from build123d import *

# Parameters (mm, degrees)
F0_R     = 16.25
F1_DEPTH = 9
F2_D     = 3.2
F2_DEPTH = 40


with BuildPart() as f1:
    # F0 (on Top) → F1 (new body)
    with BuildSketch(Plane.XY):
        with BuildLine():
            ThreePointArc((13.85, -17.413788), (20.040272, -9.666954), (22.25, 0))
            ThreePointArc((22.25, 0), (22.075626, 2.780148), (21.555238, 5.51672))
            Line((21.555238, 5.51672), (19.324579, 4.228848))
            Line((19.324579, 4.228848), (13.324579, 14.621152))
            Line((13.324579, 14.621152), (15.555238, 15.909024))
            ThreePointArc((15.555238, 15.909024), (14.721858, 16.683207), (13.85, 17.413788))
            Line((13.85, 17.413788), (-13.85, 17.413788))
            ThreePointArc((-13.85, 17.413788), (-22.25, 0), (-13.85, -17.413788))
            Line((-13.85, -17.413788), (13.85, -17.413788))
        make_face()
        Circle(F0_R, mode=Mode.SUBTRACT)
        with BuildLine():
            ThreePointArc((-8.031189, -20.75), (-11.067032, -19.302417), (-13.85, -17.413788))
            Line((-13.85, -17.413788), (-13.85, -28.75))
            Line((-13.85, -28.75), (-10.25, -28.75))
            Line((-10.25, -28.75), (-10.25, -20.75))
            Line((-10.25, -20.75), (-8.031189, -20.75))
        make_face()
        with BuildLine():
            ThreePointArc((8.031189, -20.75), (11.067032, -19.302417), (13.85, -17.413788))
            Line((13.85, -17.413788), (-13.85, -17.413788))
            ThreePointArc((-13.85, -17.413788), (-11.067032, -19.302417), (-8.031189, -20.75))
            Line((-8.031189, -20.75), (8.031189, -20.75))
        make_face()
        with BuildLine():
            Line((13.85, -28.75), (13.85, -17.413788))
            ThreePointArc((13.85, -17.413788), (11.067032, -19.302417), (8.031189, -20.75))
            Line((8.031189, -20.75), (10.25, -20.75))
            Line((10.25, -20.75), (10.25, -28.75))
            Line((10.25, -28.75), (13.85, -28.75))
        make_face()
        with BuildLine():
            ThreePointArc((8.031189, 20.75), (11.067032, 19.302417), (13.85, 17.413788))
            Line((13.85, 17.413788), (13.85, 28.75))
            Line((13.85, 28.75), (10.25, 28.75))
            Line((10.25, 28.75), (10.25, 20.75))
            Line((10.25, 20.75), (8.031189, 20.75))
        make_face()
        with BuildLine():
            Line((-13.85, 17.413788), (13.85, 17.413788))
            ThreePointArc((13.85, 17.413788), (11.067032, 19.302417), (8.031189, 20.75))
            Line((8.031189, 20.75), (-8.031189, 20.75))
            ThreePointArc((-8.031189, 20.75), (-11.067032, 19.302417), (-13.85, 17.413788))
        make_face()
        with BuildLine():
            Line((-13.85, 28.75), (-13.85, 17.413788))
            ThreePointArc((-13.85, 17.413788), (-11.067032, 19.302417), (-8.031189, 20.75))
            Line((-8.031189, 20.75), (-10.25, 20.75))
            Line((-10.25, 20.75), (-10.25, 28.75))
            Line((-10.25, 28.75), (-13.85, 28.75))
        make_face()
    extrude(amount=F1_DEPTH)

    # F2
    with Locations(Plane(origin=(0, 0, 0), x_dir=(1, 0, 0), z_dir=(0, 0, -1))):
        with Locations((-9.625, -16.670989), (9.625, -16.670989), (19.25, 0), (9.625, 16.670989), (-9.625, 16.670989), (-19.25, 0)):
            Hole(F2_D / 2, depth=F2_DEPTH)


solid = f1.part
The listing builds one solid part. Answer for the finished solid, in the listing's coordinates (mm). A direction names the side the tool comes from. Coordinates: 2 decimals unless noted, no trailing zeros. Write each loop counter-clockwise with the first axis right and the second up, starting at its lowest first coordinate (ties: lowest second). Pieces come first, ordered by that corner, then holes. Notation, with made-up numbers: (50, 48) - (96, 48) arc R14 cw to (96, 63) - close; hole circle Ø3 at (49.5, 74.5). An arc over 180 degrees is marked (long way). Put each result on its own line as item: value.
1. The part is cut by section A-A on x = 0. Give the vertices of the cut face in (y, z), plus the area to 3 significant figures.
Answer sheet:
outline: (-20.75, 0) - (-16.25, 0) - (-16.25, 9) - (-20.75, 9) - close; (16.25, 0) - (20.75, 0) - (20.75, 9) - (16.25, 9) - close
area: 81.0 mm^2
2. The part is cut by section C-C on z = 7.5. Give the vertices of the cut face in (x, y) (3 decimals).
Answer sheet:
outline: (-13.85, -28.75) - (-10.25, -28.75) - (-10.25, -20.75) - (10.25, -20.75) - (10.25, -28.75) - (13.85, -28.75) - (13.85, -17.414) arc R22.25 ccw to (22.25, 0) arc R22.25 ccw to (21.555, 5.517) - (19.325, 4.229) - (13.325, 14.621) - (15.555, 15.909) arc R22.25 ccw to (13.85, 17.414) - (13.85, 28.75) - (10.25, 28.75) - (10.25, 20.75) - (-10.25, 20.75) - (-10.25, 28.75) - (-13.85, 28.75) - (-13.85, 17.414) arc R22.25 ccw to (-13.85, -17.414) - close; hole circle Ø3.2 at (-19.25, 0); hole circle Ø32.5 at (0, 0); hole circle Ø3.2 at (-9.625, -16.671); hole circle Ø3.2 at (-9.625, 16.671); hole circle Ø3.2 at (9.625, -16.671); hole circle Ø3.2 at (9.625, 16.671); hole circle Ø3.2 at (19.25, 0)
3. A tool of negligible diameter and unlimited length cuts with its end or side. For faces 4 (the face through (-13.85, 23, 4)), 5 (the face through (13.85, 23, 4)), 6 (the face through (10.25, -25, 4)), from which of +Z, -Z, +X, -X, +Y, -Y can it reach the whole face along a straight path? Write none if from no direction.
Answer sheet:
face 4: +Z, -Z, -X, +Y
face 5: +Z, -Z, +X, +Y
face 6: +Z, -Z, -Y
4. Find the intervals of material crossed by line 1 along X through (y, z) = (26, 6); line 2 along X through (y, z) = (5, 4.75); line 3 along Y through (x, z) = (10, 3.75), in increasing order. Write a range as from..to.
Answer sheet:
line 1: x = -13.85..-10.25, 10.25..13.85
line 2: x = -21.68..-15.46, 15.46..18.88, 20.66..21.68
line 3: y = -20.75..-18.23, -15.12..-12.81, 12.81..15.12, 18.23..20.75
5. The part is cut by section B-B on y = -9. Give the vertices of the cut face in (x, z).
Answer sheet:
outline: (-20.35, 0) - (-13.53, 0) - (-13.53, 9) - (-20.35, 9) - close; (13.53, 0) - (20.35, 0) - (20.35, 9) - (13.53, 9) - close
6. Flat-ended cylindrical pins translate along their axes: pin 1 Ø6 at (x, y) = (-6, -18.5) entering from -Z; pin 2 Ø2.5 at (x, y) = (-9.62, -16.67) entering from -Z; pin 3 Ø2.5 at (y, z) = (-22.5, 6.5) entering from +X; pin 4 Ø4 at (x, z) = (16, 4.5) entering from -Y. Find the tip coordinate at first contact, or state that the pin passes through.
Answer sheet:
pin 1: stops at z = 0
pin 2: passes through
pin 3: stops at x = 13.85
pin 4: stops at y = -17.29
7. Determine the mould class of faces 1 (the face through (22.08, 2.74, 4.44)), 2 (the face through (11.223, -16.741, 4.563)), 3 (the face through (19.98, -9.79, 4.44)) for opening direction Y: pulls with the +Y half, pulls with the -Y half, needs draft (parallel to the pull), parting line crosses it, or undercut.
Answer sheet:
face 1: pulls with the +Y half
face 2: undercut
face 3: pulls with the -Y half
